Geometry check sheet. Reference: the model listing, model coordinates, mm. Face numbers are marked on the shaded views. Give positions to 0.01 mm unless a question says otherwise; leave off trailing zeros. Loops run counter-clockwise (first coordinate to the right, second up) from the corner with the lowest first, then second, coordinate; pieces in that order, holes last. Notation, with made-up numbers: (88, -32) - (123, -32) arc R29 cw to (123, -11) - close; hole circle Ø1 at (22, 5). An arc over 180 degrees is marked (long way). Use a Markdown table: item, result. Add a question column.
1. Draft check along Y on the marked faces 1, 2 and 3. Enter one of: pulls with the +Y half, pulls with the -Y half, needs draft (parallel to the pull), parting line crosses it, or undercut.
2. Depth check by flat-ended pin: P1, Ø8, axis at x = -1, y = 3, coming from the -Z side; P2, Ø1, axis at y = -5, z = 9, coming from the +X side; P3, Ø5, axis at y = -9.5, z = 8, coming from the -X side. Enter the tip coordinate at first touch or a pass-through.
3. Cross-section at D-D on x = 11. Enter the section's corners in (y, z).
4. Material ranges on L1, parallel to Y at x = 0, z = 7.75 (3 decimals); L2, parallel to Y at x = 5.5, z = 3.5; L3, parallel to Z at x = -2.5, y = -14.5, recorded low to high.
5. Cross-section at C-C on z = 11. Enter the section's corners in (x, y) (3 decimals).
6. Cross-section at A-A on x = 0. Enter the section's corners in (y, z) (3 decimals).
from build123d import *

# Parameters (mm, degrees)
F0_R     = 12.128182
F1_DEPTH = 12.7
F2_R     = 9.525
F3_DEPTH = 12.701
F2_R_2   = 17.465404
F2_R_3   = 12.128182
F4_DEPTH = 2.54


with BuildPart() as f1:
    # F0 (on Top) → F1 (new body)
    with BuildSketch(Plane.XY):
        Circle(F0_R)
    extrude(amount=F1_DEPTH)

    # F2 (on face) → F3 (cut, through all)
    with BuildSketch(Plane.XY.offset(12.7)):
        Circle(F2_R)
    extrude(amount=-F3_DEPTH, mode=Mode.SUBTRACT)

    # F2 (on face) → F4 (join)
    with BuildSketch(Plane.XY.offset(12.7)):
        Circle(F2_R_2)
        Circle(F2_R_3, mode=Mode.SUBTRACT)
    extrude(amount=-F4_DEPTH)


solid = f1.part
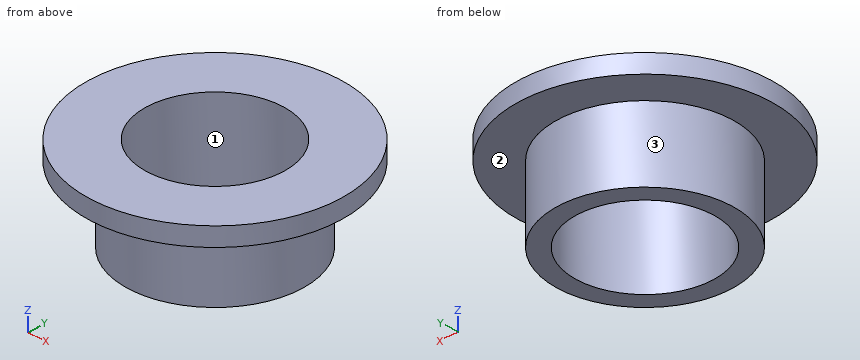
Values found:
| question | item | result |
|---|---|---|
| 1 | face 1 | undercut |
| 1 | face 2 | needs draft |
| 1 | face 3 | parting line crosses it |
| 2 | P1 | passes through |
| 2 | P2 | stops at x = 11.26 |
| 2 | P3 | stops at x = -15.4 |
| 3 | outline | (-13.57, 10.16) - (-5.11, 10.16) - (-5.11, 0) - (5.11, 0) - (5.11, 10.16) - (13.57, 10.16) - (13.57, 12.7) - (-13.57, 12.7) - close |
| 4 | L1 | y = -12.128 to -9.525, 9.525 to 12.128 |
| 4 | L2 | y = -10.81 to -7.78, 7.78 to 10.81 |
| 4 | L3 | z = 10.16 to 12.7 |
| 5 | outline | circle Ø34.931 at (0, 0); hole circle Ø19.05 at (0, 0) |
| 6 | outline | (-17.465, 10.16) - (-12.128, 10.16) - (-12.128, 0) - (-9.525, 0) - (-9.525, 12.7) - (-17.465, 12.7) - close; (9.525, 0) - (12.128, 0) - (12.128, 10.16) - (17.465, 10.16) - (17.465, 12.7) - (9.525, 12.7) - close |
